```python
from build123d import *

# Parameters (mm, degrees)
SKETCH1_R           = 0.5
BOSS_EXTRUDE1_DEPTH = 0.8


with BuildPart() as part:
    # Sketch1 → Boss-Extrude1 (new, symmetric)
    with BuildSketch(Plane(origin=(0, 0, 0), x_dir=(1, 0, 0), z_dir=(0, 1, 0))):
        Polygon((-19.05, -9.398), (-18.288, -10.16), (19.05, -10.16), (19.05, 10.16), (-18.288, 10.16), (-19.05, 9.398), align=None)
        with Locations(Location((-17.78, -8.89, 0), (0, 0, 270))):
            Circle(SKETCH1_R, mode=Mode.SUBTRACT)
        with Locations(Location((15.24, -8.89, 0), (0, 0, 270))):
            Circle(SKETCH1_R, mode=Mode.SUBTRACT)
        with Locations(Location((17.78, -8.89, 0), (0, 0, 270))):
            Circle(SKETCH1_R, mode=Mode.SUBTRACT)
        with Locations(Location((15.24, -6.35, 0), (0, 0, 270))):
            Circle(SKETCH1_R, mode=Mode.SUBTRACT)
        with Locations(Location((17.78, -6.35, 0), (0, 0, 270))):
            Circle(SKETCH1_R, mode=Mode.SUBTRACT)
        with Locations(Location((15.24, -3.81, 0), (0, 0, 270))):
            Circle(SKETCH1_R, mode=Mode.SUBTRACT)
        with Locations(Location((17.78, -3.81, 0), (0, 0, 270))):
            Circle(SKETCH1_R, mode=Mode.SUBTRACT)
        with Locations(Location((15.24, -1.27, 0), (0, 0, 270))):
            Circle(SKETCH1_R, mode=Mode.SUBTRACT)
        with Locations(Location((17.78, -1.27, 0), (0, 0, 270))):
            Circle(SKETCH1_R, mode=Mode.SUBTRACT)
        with Locations(Location((-17.78, 8.89, 0), (0, 0, 270))):
            Circle(SKETCH1_R, mode=Mode.SUBTRACT)
        with Locations(Location((15.24, 1.27, 0), (0, 0, 270))):
            Circle(SKETCH1_R, mode=Mode.SUBTRACT)
        with Locations(Location((17.78, 1.27, 0), (0, 0, 270))):
            Circle(SKETCH1_R, mode=Mode.SUBTRACT)
        with Locations(Location((15.24, 3.81, 0), (0, 0, 270))):
            Circle(SKETCH1_R, mode=Mode.SUBTRACT)
        with Locations(Location((17.78, 3.81, 0), (0, 0, 270))):
            Circle(SKETCH1_R, mode=Mode.SUBTRACT)
        with Locations(Location((15.24, 6.35, 0), (0, 0, 270))):
            Circle(SKETCH1_R, mode=Mode.SUBTRACT)
        with Locations(Location((17.78, 6.35, 0), (0, 0, 270))):
            Circle(SKETCH1_R, mode=Mode.SUBTRACT)
        with Locations(Location((15.24, 8.89, 0), (0, 0, 270))):
            Circle(SKETCH1_R, mode=Mode.SUBTRACT)
        with Locations(Location((17.78, 8.89, 0), (0, 0, 270))):
            Circle(SKETCH1_R, mode=Mode.SUBTRACT)
    extrude(amount=BOSS_EXTRUDE1_DEPTH, both=True)


solid = part.part
```
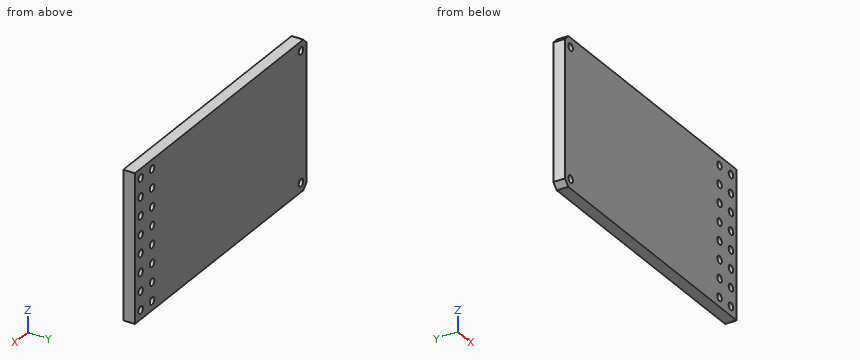
Geometry: final body of the model. Coordinates: model frame, mm. Round coordinates to 2 decimals unless told otherwise and drop trailing zeros. Write each loop counter-clockwise with the first axis right and the second up, starting at its lowest first coordinate (ties: lowest second). Pieces come first, ordered by that corner, then holes. Notation, with made-up numbers: (-25, 30.5) -> (11, 30.5) arc R8 cw to (11, 44.5) -> close; hole circle Ø7 at (28.25, 5.25). An arc over 180 degrees is marked (long way). Return JSON: item names as keys, results as strings.
Q1. Section D-D on z = -1.27. Return the cut outline in (x, y), and give its area (3 significant figures).
From the geometry:
{"outline": "(-19.05, -0.8) -> (14.74, -0.8) -> (14.74, 0.8) -> (-19.05, 0.8) -> close; (15.74, -0.8) -> (17.28, -0.8) -> (17.28, 0.8) -> (15.74, 0.8) -> close; (18.28, -0.8) -> (19.05, -0.8) -> (19.05, 0.8) -> (18.28, 0.8) -> close", "area": "57.8 mm2"}
Q2. Section B-B on y = 0. Give the number of separate pieces and of enclosed holes in the cut face, and give its area (3 significant figures).
From the geometry:
{"separate pieces": "1", "enclosed holes": "18", "area": "759 mm2"}
Q3. Section C-C on x = -17.78. Return the cut outline in (y, z), and give its area (3 significant figures).
From the geometry:
{"outline": "(-0.8, -10.16) -> (0.8, -10.16) -> (0.8, -9.39) -> (-0.8, -9.39) -> close; (-0.8, -8.39) -> (0.8, -8.39) -> (0.8, 8.39) -> (-0.8, 8.39) -> close; (-0.8, 9.39) -> (0.8, 9.39) -> (0.8, 10.16) -> (-0.8, 10.16) -> close", "area": "29.3 mm2"}
Q4. Ray query, line 1 (X direction, y = -0.4, z = -8.89); line 2 (X direction, y = 0.05, z = 3.81); line 3 (X direction, y = 0.3, z = 9). Return the intervals inside material, ascending.
From the geometry:
{"line 1": "-19.05 to -18.28, -17.28 to 14.74, 15.74 to 17.28, 18.28 to 19.05", "line 2": "-19.05 to 14.74, 15.74 to 17.28, 18.28 to 19.05", "line 3": "-19.05 to -18.27, -17.29 to 14.75, 15.73 to 17.29, 18.27 to 19.05"}
Q5. Section A-A on z = 8.89. Return the cut outline in (x, y), and give its area (3 significant figures).
From the geometry:
{"outline": "(-19.05, -0.8) -> (-18.28, -0.8) -> (-18.28, 0.8) -> (-19.05, 0.8) -> close; (-17.28, -0.8) -> (14.74, -0.8) -> (14.74, 0.8) -> (-17.28, 0.8) -> close; (15.74, -0.8) -> (17.28, -0.8) -> (17.28, 0.8) -> (15.74, 0.8) -> close; (18.28, -0.8) -> (19.05, -0.8) -> (19.05, 0.8) -> (18.28, 0.8) -> close", "area": "56.2 mm2"}
